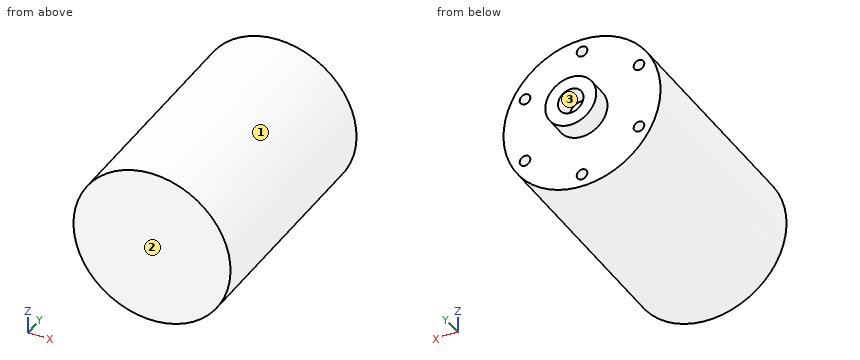
```python
from build123d import *

# Parameters (mm, degrees)
SKETCH1_R                 = 18.5
BOSS_EXTRUDE1_DEPTH       = 55.8
SKETCH2_R                 = 6
BOSS_EXTRUDE2_DEPTH       = 5
M3X0_5_TAPPED_HOLE1_D     = 2.5
M3X0_5_TAPPED_HOLE1_DEPTH = 10.67
M3X0_5_TAPPED_HOLE1_TIP   = 0.751075774
SKETCH8_R                 = 3
CUT_EXTRUDE1_DEPTH        = 5


with BuildPart() as part:
    # Sketch1 → Boss-Extrude1 (new body)
    with BuildSketch(Plane(origin=(0, 0, 0), x_dir=(1, 0, 0), z_dir=(0, 1, 0))):
        with Locations(Location((0, 0, 0), (0, 0, 270))):
            Circle(SKETCH1_R)
    extrude(amount=BOSS_EXTRUDE1_DEPTH)

    # Sketch2 → Boss-Extrude2 (add)
    with BuildSketch(Plane(origin=(0, 55.8, 0), x_dir=(1, 0, 0), z_dir=(0, 1, 0))):
        with Locations(Location((0, 0, 0), (0, 0, 270))):
            Circle(SKETCH2_R)
    extrude(amount=BOSS_EXTRUDE2_DEPTH)

    # M3x0.5 Tapped Hole1
    with Locations(Plane(origin=(0, 55.8, 0), x_dir=(1, 0, 0), z_dir=(0, 1, 0))):
        with Locations((0, 15.5), (13.423393759, 7.75), (13.423393759, -7.75), (0, -15.5), (-13.423393759, -7.75), (-13.423393759, 7.75)):
            Hole(M3X0_5_TAPPED_HOLE1_D / 2, depth=M3X0_5_TAPPED_HOLE1_DEPTH)
            with Locations((0, 0, -(M3X0_5_TAPPED_HOLE1_DEPTH + M3X0_5_TAPPED_HOLE1_TIP / 2))):  # 118° drill point
                Cone(0, M3X0_5_TAPPED_HOLE1_D / 2, M3X0_5_TAPPED_HOLE1_TIP, mode=Mode.SUBTRACT)

    # Sketch8 → Cut-Extrude1 (cut)
    with BuildSketch(Plane(origin=(0, 60.8, 0), x_dir=(1, 0, 0), z_dir=(0, 1, 0))):
        with Locations(Location((0, 0, 0), (0, 0, 270))):
            Circle(SKETCH8_R)
    extrude(amount=-CUT_EXTRUDE1_DEPTH, mode=Mode.SUBTRACT)


solid = part.part
```
Work out the finished part from the listing and answer in its coordinate system (mm). Face numbers are marked on the shaded views. Give positions to 0.01 mm unless a question says otherwise; leave off trailing zeros. Order: outer loops, then holes, each group sorted by start corner. A loop starts at its lowest first (then second) coordinate and runs counter-clockwise, first axis right, second up.
1. Section A-A, the plane z = 0 is taken. Determine the outline of the cut face in (x, y), and give its area (3 significant figures).
Result sheet:
outline: (-18.5, 0) - (18.5, 0) - (18.5, 55.8) - (6, 55.8) - (6, 60.8) - (3, 60.8) - (3, 55.8) - (-3, 55.8) - (-3, 60.8) - (-6, 60.8) - (-6, 55.8) - (-18.5, 55.8) - close
area: 2,090 mm2
2. Section C-C, the plane y = 21 is taken. Determine the outline of the cut face in (x, z).
Result sheet:
outline: circle Ø37 at (0, 0)
3. Straight lines are drawn through the part: L1, parallel to X at y = 51.5, z = 7.75; L2, parallel to X at y = 53, z = -7; L3, parallel to Y at x = -16.5, z = 1. For each, find the intervals that lie inside material, in ascending order.
Result sheet:
L1: x = -16.8 to -14.67, -12.17 to 12.17, 14.67 to 16.8
L2: x = -17.12 to -14.42, -12.42 to 12.42, 14.42 to 17.12
L3: y = 0 to 55.8
4. Each of these flat-tipped pins is pushed along its axis until it touches: P1, Ø1.8, axis at x = 1.5, z = 0, coming from the +Y side; P2, Ø2, axis at x = 13.42, z = -7.75, coming from the +Y side; P3, Ø4, axis at y = 46.5, z = 0.5, coming from the -X side. Where does it stop, or does it pass through?
Result sheet:
P1: stops at y = 55.8
P2: stops at y = 44.98
P3: stops at x = -18.5
5. The mould has two halves that part along Z. Classify the marked faces 1, 2 and 3: released by +Z, released by -Z, zero draft, split by the parting line, or undercut.
Result sheet:
face 1: split by the parting line
face 2: zero draft
face 3: undercut
6. Section D-D, the plane x = 5 is taken. Determine the outline of the cut face in (y, z).
Result sheet:
outline: (0, -17.81) - (55.8, -17.81) - (55.8, -3.32) - (60.8, -3.32) - (60.8, 3.32) - (55.8, 3.32) - (55.8, 17.81) - (0, 17.81) - close
7. Section B-B, the plane x = -4.5 is taken. Determine the outline of the cut face in (y, z).
Result sheet:
outline: (0, -17.94) - (55.8, -17.94) - (55.8, -3.97) - (60.8, -3.97) - (60.8, 3.97) - (55.8, 3.97) - (55.8, 17.94) - (0, 17.94) - close
